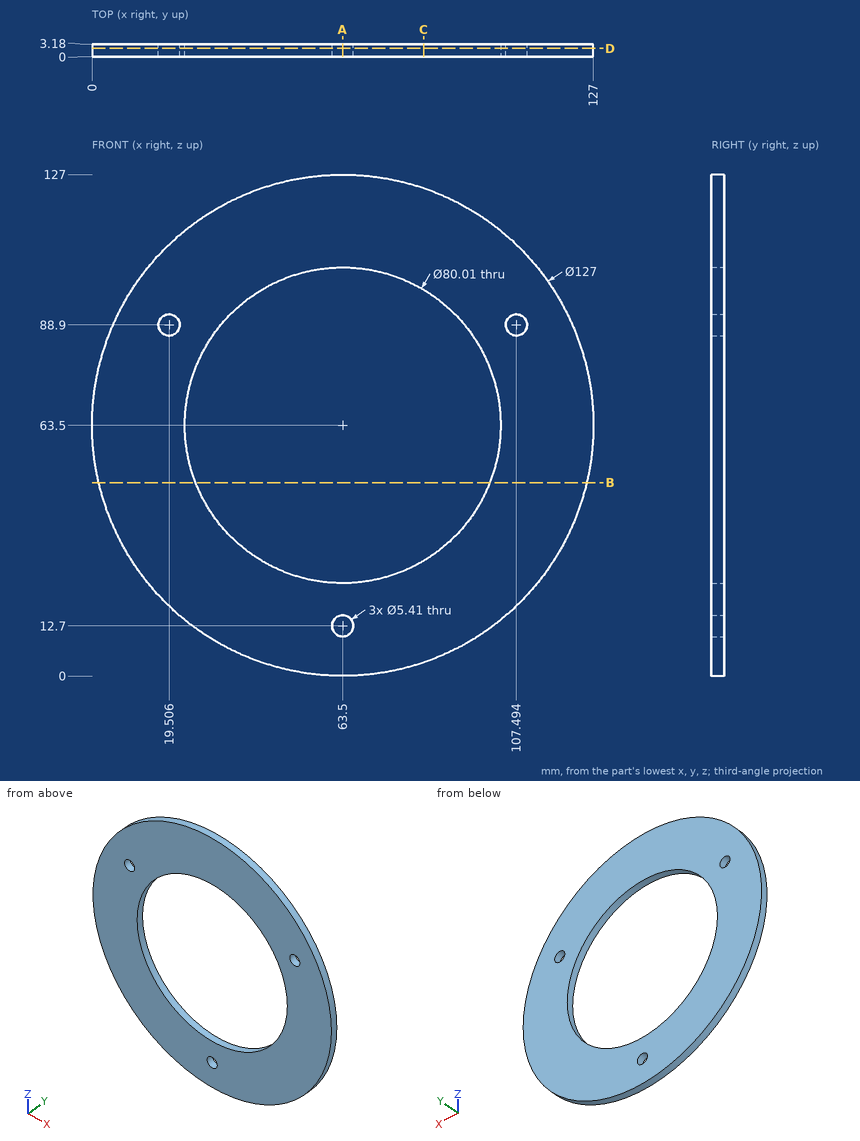
Answer from the drawing. Dimensions are ordinates in mm from the lowest x, y and z of the part. Coordinates: 2 decimals unless noted, no trailing zeros. Write each loop counter-clockwise with the first axis right and the second up, starting at its lowest first coordinate (ties: lowest second). Pieces come first, ordered by that corner, then holes. Notation, with made-up numbers: (-6, -25) - (10, -25) arc R19 ccw to (10, 10) - close; hole circle Ø9 at (-1.5, 59). An arc over 180 degrees is marked (long way). Return JSON: item names as keys, results as strings.
1. The part is cut by section B-B on z = 49. Determine the outline of the cut face in (x, y) (1 decimal).
Final values:
{"outline": "(1.7, 0) - (26.2, 0) - (26.2, 3.2) - (1.7, 3.2) - close; (100.8, 0) - (125.3, 0) - (125.3, 3.2) - (100.8, 3.2) - close"}
2. Consider line 1 along Z through (x, y) = (63.5, 1.7) (1 decimal); line 2 along X through (y, z) = (1.8, 88.9); line 3 along X through (y, z) = (0.8, 63.5) (3 decimals). Determine where each line is inside the solid, lowest interval first.
Final values:
{"line 1": "0 to 10, 15.4 to 23.5, 103.5 to 127", "line 2": "5.3 to 16.8, 22.21 to 32.59, 94.41 to 104.79, 110.2 to 121.7", "line 3": "0 to 23.495, 103.505 to 127"}
3. This flat-tipped pin is pushed along its axis until it touches: pin 1 Ø3 at (x, z) = (107.49, 88.9) entering from +Y. Where does it stop, or does it pass through?
Final values:
{"pin 1": "through"}
4. The part is cut by section D-D on y = 2.05. Determine the outline of the cut face in (x, z) (1 decimal), then the cut area to 3 significant figures.
Final values:
{"outline": "circle Ø127 at (63.5, 63.5); hole circle Ø5.4 at (19.5, 88.9); hole circle Ø80 at (63.5, 63.5); hole circle Ø5.4 at (63.5, 12.7); hole circle Ø5.4 at (107.5, 88.9)", "area": "7,570 mm^2"}
5. The part is cut by section C-C on x = 84. Determine the outline of the cut face in (y, z), then the cut area to 3 significant figures.
Final values:
{"outline": "(0, 3.4) - (3.18, 3.4) - (3.18, 29.15) - (0, 29.15) - close; (0, 97.85) - (3.18, 97.85) - (3.18, 123.6) - (0, 123.6) - close", "area": "164 mm^2"}
6. The part is cut by section A-A on x = 63.5. Determine the outline of the cut face in (y, z) (1 decimal), then the cut area to 3 significant figures.
Final values:
{"outline": "(0, 0) - (3.2, 0) - (3.2, 10) - (0, 10) - close; (0, 15.4) - (3.2, 15.4) - (3.2, 23.5) - (0, 23.5) - close; (0, 103.5) - (3.2, 103.5) - (3.2, 127) - (0, 127) - close", "area": "132 mm^2"}
